Geometry: final body of the model. Coordinates: model frame, mm. A direction names the side the tool comes from. Coordinates: 2 decimals unless noted, no trailing zeros. Write each loop counter-clockwise with the first axis right and the second up, starting at its lowest first coordinate (ties: lowest second). Pieces come first, ordered by that corner, then holes. Notation, with made-up numbers: (-37.75, -25.75) - (5.25, -25.75) arc R19 cw to (5.25, -3.75) - close; hole circle Ø7 at (-10.5, 60). An arc over 180 degrees is marked (long way). Put each result on its own line as item: value.
```python
from build123d import *

# Parameters (mm, degrees)
F1_DEPTH = 3
F2_R     = 5
F3_R     = 15
F4_R     = 15
F5_R     = 15


with BuildPart() as f1:
    # F0 (on Front) → F1 (new body)
    with BuildSketch(Plane.XZ):
        with BuildLine():
            Line((0, 145), (0, 0))
            Line((0, 0), (25, 0))
            Line((25, 0), (25, 75))
            Line((25, 75), (100, 75))
            Line((100, 75), (100, 145))
            ThreePointArc((100, 145), (98.535534, 148.535534), (95, 150))
            Line((95, 150), (5, 150))
            ThreePointArc((5, 150), (1.464466, 148.535534), (0, 145))
        make_face()
    extrude(amount=F1_DEPTH)

    # F2
    f2_edges = [f1.edges().sort_by_distance(p)[0] for p in [
        (0, -1.5, 0),
    ]]
    fillet(f2_edges, radius=F2_R)

    # F3
    f3_edges = [f1.edges().sort_by_distance(p)[0] for p in [
        (100, -1.5, 75),
    ]]
    fillet(f3_edges, radius=F3_R)

    # F4
    f4_edges = [f1.edges().sort_by_distance(p)[0] for p in [
        (25, -1.5, 0),
    ]]
    fillet(f4_edges, radius=F4_R)

    # F5
    f5_edges = [f1.edges().sort_by_distance(p)[0] for p in [
        (25, -1.5, 75),
    ]]
    fillet(f5_edges, radius=F5_R)


solid = f1.part
```
1. Set-up query: faces 1 (the flat face through (25, -1, 37)), 2 (the cylindrical face through (1, -2, 2)). Return all of +Z, -Z, +X, -X, +Y, -Y with unobstructed straight access to the full face (end or side cutting, diameter ignored); none if empty.
Answer below:
face 1: -Z, +X, +Y, -Y
face 2: -Z, -X, +Y, -Y
2. Section query C-C (x = 54). Return loops of the section in (y, z).
Answer below:
outline: (-3, 75) - (0, 75) - (0, 150) - (-3, 150) - close
3. Pin query (flat end, axial travel): pin 1 Ø1.5 at (x, y) = (55.5, -1) entering from -Z; pin 2 Ø1.5 at (x, y) = (22, -1.5) entering from -Z. Return the tip coordinate at first contact, or that it passes through.
Answer below:
pin 1: stops at z = 75
pin 2: stops at z = 5.08
4. Ray query, probe 1 along Z at (x, y) = (65, -0.65); probe 2 along X at (y, z) = (-0.7, 36.5); probe 3 along Z at (x, y) = (33.5, -1). Return the intervals inside material, ascending. Write a range as from..to.
Answer below:
probe 1: z = 75..150
probe 2: x = 0..25
probe 3: z = 73.52..150
5. Section query B-B (z = 27.5). Return loops of the section in (x, y), then the cut area to 3 significant figures.
Answer below:
outline: (0, -3) - (25, -3) - (25, 0) - (0, 0) - close
area: 75.0 mm²
6. Section query A-A (y = -1.6). Return loops of the section in (x, z).
Answer below:
outline: (0, 5) arc R5 ccw to (5, 0) - (10, 0) arc R15 ccw to (25, 15) - (25, 60) arc R15 cw to (40, 75) - (85, 75) arc R15 ccw to (100, 90) - (100, 145) arc R5 ccw to (95, 150) - (5, 150) arc R5 ccw to (0, 145) - close
